The listing builds one solid part. Answer for the finished solid, in the listing's coordinates (mm). Give positions to 0.01 mm unless a question says otherwise; leave off trailing zeros. Loops run counter-clockwise (first coordinate to the right, second up) from the corner with the lowest first, then second, coordinate; pieces in that order, holes last. Notation, with made-up numbers: (-25, 62.25) - (25, 62.25) arc R19 cw to (25, 83.25) - close; hole circle Ø5 at (30, 40.5). An arc over 180 degrees is marked (long way). Write each question's results on one line, items separated by ' | '.
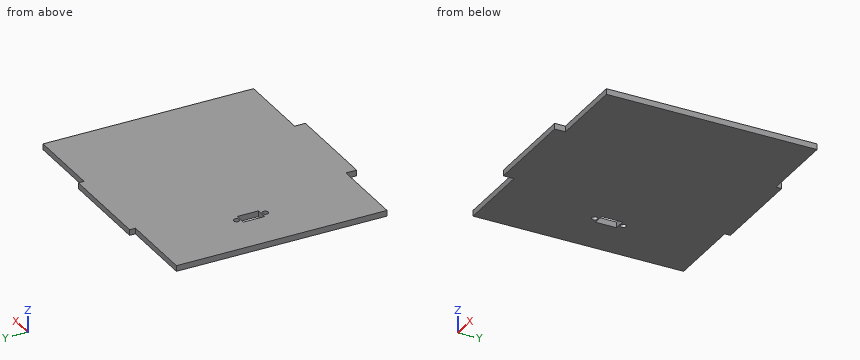
Autodesk Inventor part; units mm, degrees
ref_plane "YZ Plane" through (0, 0, 0) normal (1, 0, 0) x (0, 1, 0)
ref_plane "XZ Plane" through (0, 0, 0) normal (0, 1, 0) x (-1, 0, 0)
ref_plane "XY Plane" through (0, 0, 0) normal (0, 0, 1) x (1, 0, 0)
sketch "Sketch1" plane through (0, 0, 0) normal (0, 0, 1) x (1, 0, 0)
  line L0 (-70.131, 85.6788) -> (-70.131, -24.3212)
  line L1 (-70.131, -24.3212) -> (-30.131, -24.3212)
  line L2 (-30.131, -24.3212) -> (-30.131, -29.9212)
  line L3 (-30.131, -29.9212) -> (19.869, -29.9212)
  line L4 (19.869, -29.9212) -> (19.869, -24.3212)
  line L5 (19.869, -24.3212) -> (59.869, -24.3212)
  line L6 (59.869, -24.3212) -> (59.869, 85.6788)
  line L7 (59.869, 85.6788) -> (19.869, 85.6788)
  line L8 (19.869, 85.6788) -> (19.869, 88.6788)
  line L9 (19.869, 88.6788) -> (-30.131, 88.6788)
  line L10 (-30.131, 88.6788) -> (-30.131, 85.6788)
  line L11 (-30.131, 85.6788) -> (-70.131, 85.6788)
  line L12 (-5.131, 88.6788) -> (-5.131, -29.9212) construction
  line L13 (-48.5521, 39.0524) -> (-48.5521, 28.0524)
  line L14 (-48.5521, 28.0524) -> (-42.5521, 28.0524)
  line L15 (-42.5521, 28.0524) -> (-42.5521, 39.0524)
  line L16 (-42.5521, 39.0524) -> (-48.5521, 39.0524)
  circle A0 centre (-45.5521, 41.0524) radius 1.5
  circle A1 centre (-45.5521, 26.0524) radius 1.5
  line L17 (-45.5521, 26.0524) -> (-45.5521, 41.0524) construction
  point P0 (0, 0)
  dimension "d0" = 130
  dimension "d1" = 110
  dimension "d2" = 50
  dimension "d3" = 50
  dimension "d4" = 11
  dimension "d5" = 6
  dimension "d6" = 3
  dimension "d7" = 2
  dimension "d8" = 3
  dimension "d9" = 2
  dimension "d12" = 3
  dimension "d13" = 5.6
extrude "Extrusion1" add sketch "Sketch1" along normal blind 3
properties part number "BackWallV2"
Item 1: Flat-ended cylindrical pins translate along their axes: P1, Ø1.5, axis at y = -26, z = 1.5, coming from the -X side; P2, Ø1.5, axis at x = -46.5, z = 1, coming from the -Y side; P3, Ø1.5, axis at y = 86.5, z = 1.5, coming from the +X side. Find the tip coordinate at first contact, or state that the pin passes through.
Values found:
P1: stops at x = -30.13 | P2: stops at y = -24.32 | P3: stops at x = 19.87
Item 2: Find the intervals of material crossed by line 1 along X through (y, z) = (41, 2.1); line 2 along Y through (x, z) = (-44, 0.2); line 3 along X through (y, z) = (30, 0.4), in increasing order. Write a range as [from, to].
Values found:
line 1: x = [-70.13, -47.05], [-44.05, 59.87] | line 2: y = [-24.32, 28.05], [39.05, 85.68] | line 3: x = [-70.13, -48.55], [-42.55, 59.87]
Item 3: A cutting plane is placed at A-A, the plane z = 1. Determine the outline of the cut face in (x, y), plus the area to 3 significant figures.
Values found:
outline: (-70.13, -24.32) - (-30.13, -24.32) - (-30.13, -29.92) - (19.87, -29.92) - (19.87, -24.32) - (59.87, -24.32) - (59.87, 85.68) - (19.87, 85.68) - (19.87, 88.68) - (-30.13, 88.68) - (-30.13, 85.68) - (-70.13, 85.68) - close; hole (-48.55, 28.05) - (-42.55, 28.05) - (-42.55, 39.05) - (-48.55, 39.05) - close; hole circle Ø3 at (-45.55, 26.05); hole circle Ø3 at (-45.55, 41.05) | area: 14,600 mm²
